Build history of the part. All positions in model axes, mm. Give positions to 0.01 mm unless a question says otherwise; leave off trailing zeros. Write each loop counter-clockwise with the first axis right and the second up, starting at its lowest first coordinate (ties: lowest second). Pieces come first, ordered by that corner, then holes.
from build123d import *

# Parameters (mm, degrees)
F0_R     = 10
F1_DEPTH = 2
F3_DEPTH = 2.001


with BuildPart() as f1:
    # F0 (on Front) → F1 (new body)
    with BuildSketch(Plane.XZ):
        Circle(F0_R)
    extrude(amount=F1_DEPTH)

    # F2 (on face) → F3 (cut, through all)
    with BuildSketch(Plane.XZ.offset(2)):
        with BuildLine():
            ThreePointArc((4.795326069, 5.0994948663), (4.3154664556, 2.525222618), (6.7947838404, 1.6825315934))
            ThreePointArc((6.7947838404, 1.6825315934), (6.0416530379, 3.5353116652), (4.795326069, 5.0994948663))
        make_face()
        with BuildLine():
            ThreePointArc((4.795326069, 5.0994948663), (6.0416530379, 3.5353116652), (6.7947838404, 1.6825315934))
            ThreePointArc((6.7947838404, 1.6825315934), (7.700909137, 2.4186786917), (8.0416530379, 3.5353116652))
            ThreePointArc((8.0416530379, 3.5353116652), (6.9097964771, 5.3370682994), (4.795326069, 5.0994948663))
        make_face()
        with BuildLine():
            ThreePointArc((7.8100628501, -3.9042502068), (7.5032590313, -2.8397847578), (6.6769761581, -2.1019013736))
            ThreePointArc((6.6769761581, -2.1019013736), (5.8100628501, -3.9042502068), (4.4688586973, -5.3878847374))
            ThreePointArc((4.4688586973, -5.3878847374), (6.6217252474, -5.7321463069), (7.8100628501, -3.9042502068))
        make_face()
        with BuildLine():
            ThreePointArc((4.4688586973, -5.3878847374), (5.8100628501, -3.9042502068), (6.6769761581, -2.1019013736))
            ThreePointArc((6.6769761581, -2.1019013736), (4.150044893, -2.7887501477), (4.4688586973, -5.3878847374))
        make_face()
        with BuildLine():
            ThreePointArc((-1.9794866372, 6.7142857143), (0, 5), (1.9794866372, 6.7142857143))
            ThreePointArc((1.9794866372, 6.7142857143), (0, 7), (-1.9794866372, 6.7142857143))
        make_face()
        with BuildLine():
            ThreePointArc((-1.9794866372, 6.7142857143), (0, 7), (1.9794866372, 6.7142857143))
            ThreePointArc((1.9794866372, 6.7142857143), (1.9948650674, 6.8567751321), (2, 7))
            ThreePointArc((2, 7), (-0.1432248679, 8.9948650674), (-1.9794866372, 6.7142857143))
        make_face()
        with BuildLine():
            ThreePointArc((2, -7), (1.9948650674, -6.8567751321), (1.9794866372, -6.7142857143))
            ThreePointArc((1.9794866372, -6.7142857143), (0, -7), (-1.9794866372, -6.7142857143))
            ThreePointArc((-1.9794866372, -6.7142857143), (-0.1432248679, -8.9948650674), (2, -7))
        make_face()
        with BuildLine():
            ThreePointArc((-1.9794866372, -6.7142857143), (0, -7), (1.9794866372, -6.7142857143))
            ThreePointArc((1.9794866372, -6.7142857143), (0, -5), (-1.9794866372, -6.7142857143))
        make_face()
        with BuildLine():
            ThreePointArc((-3.6779306672, 4.0940326499), (-3.8368770547, 4.8753914638), (-4.2884522632, 5.5325561168))
            ThreePointArc((-4.2884522632, 5.5325561168), (-5.6779306672, 4.0940326499), (-6.6039045269, 2.321302436))
            ThreePointArc((-6.6039045269, 2.321302436), (-4.6415783428, 2.3834848255), (-3.6779306672, 4.0940326499))
        make_face()
        with BuildLine():
            ThreePointArc((-6.6039045269, 2.321302436), (-5.6779306672, 4.0940326499), (-4.2884522632, 5.5325561168))
            ThreePointArc((-4.2884522632, 5.5325561168), (-7.3001965721, 5.2637562642), (-6.6039045269, 2.321302436))
        make_face()
        with BuildLine():
            ThreePointArc((-6.9101605699, -1.1178912729), (-8.1154178378, -3.891014433), (-5.1985581087, -4.6877493096))
            ThreePointArc((-5.1985581087, -4.6877493096), (-6.3119916516, -3.026344559), (-6.9101605699, -1.1178912729))
        make_face()
        with BuildLine():
            ThreePointArc((-6.9101605699, -1.1178912729), (-6.3119916516, -3.026344559), (-5.1985581087, -4.6877493096))
            ThreePointArc((-5.1985581087, -4.6877493096), (-4.5474992195, -3.9679211396), (-4.3119916516, -3.026344559))
            ThreePointArc((-4.3119916516, -3.026344559), (-5.1280021746, -1.4144609037), (-6.9101605699, -1.1178912729))
        make_face()
    extrude(amount=-F3_DEPTH, mode=Mode.SUBTRACT)


solid = f1.part
1. Saw through at C-C on z = 4.75. Give the cut face in (x, y), plus the area to 3 significant figures.
2. Drop a flat-ended pin along its axis: pin 1 (1 mm diameter, centred on y = -1.5, z = 3, fed in from -X). Give the stop position or say it passes through.
3. Saw through at D-D on x = -2.25. Give the cut face in (y, z), plus the area to 3 significant figures.
4. Saw through at B-B on x = 0. Give the cut face in (y, z), plus the area to 3 significant figures.
5. Saw through at A-A on y = -1.7. Give the cut face in (x, z), plus the area to 3 significant figures.
6. Drill centre lines: line 1 along Z through (x, y) = (-5, -0.75); line 2 along Z through (x, y) = (-1.25, -1); line 3 along X through (y, z) = (-1.65, 4.5). Where is each one in solid material? Low to high.
Outcome:
1. outline: (-8.8, -2) - (-7.57, -2) - (-7.57, 0) - (-8.8, 0) - close; (-3.79, -2) - (4.45, -2) - (4.45, 0) - (-3.79, 0) - close; (7.63, -2) - (8.8, -2) - (8.8, 0) - (7.63, 0) - close
1. area: 21.3 mm2
2. pin 1: stops at x = -9.68
3. outline: (-2, -9.74) - (0, -9.74) - (0, 9.74) - (-2, 9.74) - close
3. area: 39.0 mm2
4. outline: (-2, -10) - (0, -10) - (0, -9) - (-2, -9) - close; (-2, -5) - (0, -5) - (0, 5) - (-2, 5) - close; (-2, 9) - (0, 9) - (0, 10) - (-2, 10) - close
4. area: 24.0 mm2
5. outline: circle Ø20 at (0, 0); hole circle Ø4 at (-6.31, -3.03); hole circle Ø4 at (-5.68, 4.09); hole circle Ø4 at (0, -7); hole circle Ø4 at (0, 7); hole circle Ø4 at (5.81, -3.9); hole circle Ø4 at (6.04, 3.54)
5. area: 239 mm2
6. line 1: z = -8.66 to -4.54, -1.52 to 2.21, 5.98 to 8.66
6. line 2: z = -9.92 to -8.56, -5.44 to 5.44, 8.56 to 9.92
6. line 3: x = -8.93 to -7.64, -3.72 to 4.29, 7.79 to 8.93
